Part model, mm, in its own coordinate system. Coordinates: 2 decimals unless noted, no trailing zeros. Loops run counter-clockwise (first coordinate to the right, second up) from the corner with the lowest first, then second, coordinate; pieces in that order, holes last. Notation, with made-up numbers: M -27,-19.75 L 0,-19.75 A21 cw 0,9.25 Z; hole C 11,23 d1. An arc over 180 degrees is marked long. Use CSV: the item, a comma, the result in double quotes. Start each with the question number.
from build123d import *

# Parameters (mm, degrees)
SKETCH1_W               = 275.57984
SKETCH1_H               = 62.103
BOSS_EXTRUDE1_DEPTH     = 2.54
SKETCH2_W               = 25.4
SKETCH2_H               = 2.54
BOSS_EXTRUDE2_DEPTH     = 2.54
LPATTERN1_COUNT         = 5
LPATTERN1_PITCH         = 50.8
SKETCH3_W               = 2.54
SKETCH3_H               = 12.7
CUT_EXTRUDE1_DEPTH      = 142.848167157
LPATTERN3_COUNT         = 3
LPATTERN3_PITCH         = 25.4
MIRROR1_COPY_1_SKETCH_W = 2.54
MIRROR1_COPY_1_SKETCH_H = 12.7
MIRROR1_COPY_1_DEPTH    = 142.848167157
MIRROR1_COPY_2_SKETCH_W = 2.54
MIRROR1_COPY_2_SKETCH_H = 12.7
MIRROR1_COPY_2_DEPTH    = 142.848167157
SKETCH5_W               = 19.05
SKETCH5_H               = 2.54
CUT_EXTRUDE3_DEPTH      = 142.848167157
LPATTERN5_COUNT         = 8
LPATTERN5_PITCH         = 38.1


with BuildPart() as part:
    # Sketch1 → Boss-Extrude1 (new body)
    with BuildSketch(Plane.XY):
        Rectangle(SKETCH1_W, SKETCH1_H)
    extrude(amount=BOSS_EXTRUDE1_DEPTH)

    # Sketch2 → Boss-Extrude2 (add)
    with BuildSketch(Plane.XY.offset(2.54)):
        with Locations((-125.08992, 32.3215)):
            Rectangle(SKETCH2_W, SKETCH2_H)
    boss_extrude2 = extrude(amount=-BOSS_EXTRUDE2_DEPTH)

    # LPattern1: Boss-Extrude2 ×5
    with Locations(*[(i * LPATTERN1_PITCH, 0, 0) for i in range(1, LPATTERN1_COUNT)]):
        add(boss_extrude2)

    # Sketch3 → Cut-Extrude1 (cut, through all)
    with BuildSketch(Plane.XY.offset(2.54)):
        with Locations((-136.51992, -18.3515)):
            Rectangle(SKETCH3_W, SKETCH3_H)
    cut_extrude1 = extrude(amount=-CUT_EXTRUDE1_DEPTH, mode=Mode.SUBTRACT)

    # LPattern3: Cut-Extrude1 ×3
    with Locations(*[(0, i * LPATTERN3_PITCH, 0) for i in range(1, LPATTERN3_COUNT)]):
        add(cut_extrude1, mode=Mode.SUBTRACT)

    # Mirror1: Cut-Extrude1 across plane
    add(cut_extrude1.mirror(Plane(origin=(0, 0, 0), x_dir=(0, 0, 1), z_dir=(1, 0, 0))), mode=Mode.SUBTRACT)

    # Mirror1 copy 1 sketch → Mirror1 copy 1 (cut, through all)
    with BuildSketch(Plane(origin=(0, 25.4, 2.54), x_dir=(-1, 0, 0), z_dir=(0, 0, 1))):
        with Locations((-136.51992, 18.3515)):
            Rectangle(MIRROR1_COPY_1_SKETCH_W, MIRROR1_COPY_1_SKETCH_H)
    extrude(amount=-MIRROR1_COPY_1_DEPTH, mode=Mode.SUBTRACT)

    # Mirror1 copy 2 sketch → Mirror1 copy 2 (cut, through all)
    with BuildSketch(Plane(origin=(0, 50.8, 2.54), x_dir=(-1, 0, 0), z_dir=(0, 0, 1))):
        with Locations((-136.51992, 18.3515)):
            Rectangle(MIRROR1_COPY_2_SKETCH_W, MIRROR1_COPY_2_SKETCH_H)
    extrude(amount=-MIRROR1_COPY_2_DEPTH, mode=Mode.SUBTRACT)

    # Sketch5 → Cut-Extrude3 (cut, through all)
    with BuildSketch(Plane.XY.offset(2.54)):
        with Locations((-119.38508, -29.7815)):
            Rectangle(SKETCH5_W, SKETCH5_H)
    cut_extrude3 = extrude(amount=-CUT_EXTRUDE3_DEPTH, mode=Mode.SUBTRACT)

    # LPattern5: Cut-Extrude3 ×8
    with Locations(*[(i * LPATTERN5_PITCH, 0, 0) for i in range(1, LPATTERN5_COUNT)]):
        add(cut_extrude3, mode=Mode.SUBTRACT)


solid = part.part
1. Pin check, flat tips, straight feed: pin 1 (1.3 mm diameter, centred on x = 117, z = 2, fed in from +Y); pin 2 (1.3 mm diameter, centred on y = -19, z = 1, fed in from +X); pin 3 (12 mm diameter, centred on x = -14.5, y = -17, fed in from -Z); pin 4 (1.3 mm diameter, centred on y = 8.5, z = 1, fed in from -X). Stop position of each tip, or through.
2. Wall check: probe 1 along Y at (x, z) = (91, 1.5); probe 2 along Y at (x, z) = (-41.5, 1.1); probe 3 along X at (y, z) = (7, 0.95). Give the ranges that are in metal, low to high.
3. Slice it at A-A, the plane x = 8.5. List the corners of the cut face in (y, z), and give its area (3 significant figures).
4. Slice it at B-B, the plane y = -19. List the corners of the cut face in (x, z), and give its area (3 significant figures).
Found:
1,pin 1,"y = 31.05"
1,pin 2,"x = 135.25"
1,pin 3,"z = 0"
1,pin 4,"x = -135.25"
2,probe 1,"-31.05 to 31.05"
2,probe 2,"-28.51 to 31.05"
2,probe 3,"-135.25 to 135.25"
3,outline,"M -31.05,0 L 31.05,0 L 31.05,2.54 L -31.05,2.54 Z"
3,area,"158 mm^2"
4,outline,"M -135.25,0 L 135.25,0 L 135.25,2.54 L -135.25,2.54 Z"
4,area,"687 mm^2"
